The model under review builds one solid part; all positions refer to its coordinate system, in mm. Coordinates: 2 decimals unless noted, no trailing zeros. Loops run counter-clockwise (first coordinate to the right, second up) from the corner with the lowest first, then second, coordinate; pieces in that order, holes last. Notation, with made-up numbers: M 70.25,35 L 76.25,35 A19 cw 76.25,50 Z; hole C 20.25,-32 d10. An arc over 180 degrees is marked long. Write item = value, one per line. Start each with the question number.
Q1. Clearance check with flat-ended pins moving along their axes: pin 1 Ø5.5 at (x, y) = (1067.5, -9.5) entering from -Z; pin 2 Ø9 at (x, y) = (48, -6.5) entering from -Z; pin 3 Ø8 at (x, z) = (323.5, -145) entering from +Y. State where each tip first meets the part, or that it passes through.
Q2. Wall thickness on probe 1 along X at (y, z) = (-10, 0); probe 2 along Z at (x, y) = (35, -7.5); probe 3 along X at (y, z) = (-5.75, -303.5): over which ranges is each line inside the solid? List them lowest first.
Q3. Mouldability with a two-part tool opening along X and no side actions: class faces 1 (the face through (1075.143, -8.874, -470.218)), 2 (the face through (-1026.754, -8.874, -470.972)), 3 (the face through (1025.4, -8.87, -468.37)), 4 (the face through (-1074.483, -8.874, -467.698)) as released by +X, released by -X, zero draft, split by the parting line, or undercut.
Q4. We need section C-C on y = -3.25. Count the separate pieces of the cut face and the enclosed holes in it, and give its area (3 significant figures).
Q5. We need section B-B on z = -416. Give the boundary of the cut face in (x, y), and give its area (3 significant figures).
Q6. We need section A-A on x = -43. Give the boundary of the cut face in (y, z), and give its area (3 significant figures).
Q7. We need section D-D on x = 292.5. Give the boundary of the cut face in (y, z), and give its area (3 significant figures).
from build123d import *

# Parameters (mm, degrees)
F0_W     = 9
F0_H     = 432
F0_H_2   = 9
F1_DEPTH = 18


# Not quite as in the source:
# - a feature names something its author has since deleted; it is built from what else it names


with BuildPart() as f1:
    # F0 (on Front) → F1 (new body)
    with BuildSketch(Plane.XZ):
        Polygon((0, 75.8756743552), (-1100, 75.8756743552), (-1100, 66.8756743552), (-1091, 66.8756743552), (0, 66.8756743552), (1091, 66.8756743552), (1091, 75.8756743552), align=None)
        with BuildLine():
            Line((-973.3476458471, -374.1243256448), (-1054.6076226562, -374.1243256448))
            ThreePointArc((-1054.6076226562, -374.1243256448), (-1051.7483407187, -375.721921149), (-1051.265639742, -378.9614896944))
            Line((-1051.265639742, -378.9614896944), (-1098.3606008427, -558.954299013))
            ThreePointArc((-1098.3606008427, -558.954299013), (-1097.4812264988, -563.2754093644), (-1093.523436793, -565.219938755))
            Line((-1093.523436793, -565.219938755), (-1078.8076104242, -565.219938755))
            ThreePointArc((-1078.8076104242, -565.219938755), (-1076.2129629213, -564.4940239596), (-1074.371712623, -562.5270604893))
            Line((-1074.371712623, -562.5270604893), (-977.7835436484, -376.8172039105))
            ThreePointArc((-977.7835436484, -376.8172039105), (-975.94229335, -374.8502404402), (-973.3476458471, -374.1243256448))
        make_face()
        with BuildLine():
            Line((1100, 66.8756743552), (1091, 66.8756743552))
            Line((1091, 66.8756743552), (1091, -365.0378882885))
            Line((1091, -365.0378882885), (1091, -365.1243256448))
            Line((1091, -365.1243256448), (0, -365.1243256448))
            Line((0, -365.1243256448), (-1091, -365.1243256448))
            Line((-1091, -365.1243256448), (-1091, -374.1243256448))
            Line((-1091, -374.1243256448), (-1055, -374.1243256448))
            ThreePointArc((-1055, -374.1243256448), (-1054.8038113281, -374.1191399972), (-1054.6076226562, -374.1243256448))
            Line((-1054.6076226562, -374.1243256448), (-973.3476458471, -374.1243256448))
            Line((-973.3476458471, -374.1243256448), (0, -374.1243256448))
            Line((0, -374.1243256448), (973.3476458471, -374.1243256448))
            Line((973.3476458471, -374.1243256448), (1054.6076226562, -374.1243256448))
            ThreePointArc((1054.6076226562, -374.1243256448), (1054.8038113281, -374.1191399972), (1055, -374.1243256448))
            Line((1055, -374.1243256448), (1100, -374.1243256448))
            Line((1100, -374.1243256448), (1100, 66.8756743552))
        make_face()
        with Locations((-1095.5, -149.1243256448)):
            Rectangle(F0_W, F0_H)
        with Locations((-1095.5, -369.6243256448)):
            Rectangle(F0_W, F0_H_2)
        with Locations((1095.5, 71.3756743552)):
            Rectangle(F0_W, F0_H_2)
        with BuildLine():
            ThreePointArc((1051.265639742, -378.9614896944), (1051.7483407187, -375.721921149), (1054.6076226562, -374.1243256448))
            Line((1054.6076226562, -374.1243256448), (973.3476458471, -374.1243256448))
            ThreePointArc((973.3476458471, -374.1243256448), (975.94229335, -374.8502404402), (977.7835436484, -376.8172039105))
            Line((977.7835436484, -376.8172039105), (1074.371712623, -562.5270604893))
            ThreePointArc((1074.371712623, -562.5270604893), (1076.2129629213, -564.4940239596), (1078.8076104242, -565.219938755))
            Line((1078.8076104242, -565.219938755), (1093.523436793, -565.219938755))
            ThreePointArc((1093.523436793, -565.219938755), (1097.4812264988, -563.2754093644), (1098.3606008427, -558.954299013))
            Line((1098.3606008427, -558.954299013), (1051.265639742, -378.9614896944))
        make_face()
        Polygon((0, 66.8756743552), (-1091, 66.8756743552), (-1091, -365.1243256448), (0, -365.1243256448), (1091, -365.1243256448), (1091, -365.0378882885), (1091, 66.8756743552), align=None)
        with BuildLine():
            ThreePointArc((-1041, -227.1243239641), (-1037.4852813742, -218.6390425899), (-1029, -215.1243239641))
            Line((-1029, -215.1243239641), (-803, -215.1243239641))
            ThreePointArc((-803, -215.1243239641), (-794.5147186258, -218.6390425899), (-791, -227.1243239641))
            Line((-791, -227.1243239641), (-791, -303.1243256448))
            ThreePointArc((-791, -303.1243256448), (-794.5147186258, -311.609607019), (-803, -315.1243256448))
            Line((-803, -315.1243256448), (-1029, -315.1243256448))
            ThreePointArc((-1029, -315.1243256448), (-1037.4852813742, -311.609607019), (-1041, -303.1243256448))
            Line((-1041, -303.1243256448), (-1041, -227.1243239641))
        make_face(mode=Mode.SUBTRACT)
        with BuildLine():
            ThreePointArc((-118.4479668736, -227.1243239641), (-114.9332482479, -218.6390425899), (-106.4479668736, -215.1243239641))
            Line((-106.4479668736, -215.1243239641), (119.5520331264, -215.1243239641))
            ThreePointArc((119.5520331264, -215.1243239641), (128.0373145006, -218.6390425899), (131.5520331264, -227.1243239641))
            Line((131.5520331264, -227.1243239641), (131.5520331264, -303.1243256448))
            ThreePointArc((131.5520331264, -303.1243256448), (128.0373145006, -311.609607019), (119.5520331264, -315.1243256448))
            Line((119.5520331264, -315.1243256448), (-106.4479668736, -315.1243256448))
            ThreePointArc((-106.4479668736, -315.1243256448), (-114.9332482479, -311.609607019), (-118.4479668736, -303.1243256448))
            Line((-118.4479668736, -303.1243256448), (-118.4479668736, -227.1243239641))
        make_face(mode=Mode.SUBTRACT)
        with BuildLine():
            Line((791, -303.1243256448), (791, -227.1243239641))
            ThreePointArc((791, -227.1243239641), (794.5147186258, -218.6390425899), (803, -215.1243239641))
            Line((803, -215.1243239641), (1029, -215.1243239641))
            ThreePointArc((1029, -215.1243239641), (1037.4852813742, -218.6390425899), (1041, -227.1243239641))
            Line((1041, -227.1243239641), (1041, -303.1243256448))
            ThreePointArc((1041, -303.1243256448), (1037.4852813742, -311.609607019), (1029, -315.1243256448))
            Line((1029, -315.1243256448), (803, -315.1243256448))
            ThreePointArc((803, -315.1243256448), (794.5147186258, -311.609607019), (791, -303.1243256448))
        make_face(mode=Mode.SUBTRACT)
        with BuildLine():
            ThreePointArc((-1041, 4.8756749481), (-1037.4852813742, 13.3609563223), (-1029, 16.8756749481))
            Line((-1029, 16.8756749481), (-803, 16.8756749481))
            ThreePointArc((-803, 16.8756749481), (-794.5147186258, 13.3609563223), (-791, 4.8756749481))
            Line((-791, 4.8756749481), (-791, -21.1243239343))
            ThreePointArc((-791, -21.1243239343), (-794.5147186258, -29.6096053086), (-803, -33.1243239343))
            Line((-803, -33.1243239343), (-1029, -33.1243239343))
            ThreePointArc((-1029, -33.1243239343), (-1037.4852813742, -29.6096053086), (-1041, -21.1243239343))
            Line((-1041, -21.1243239343), (-1041, 4.8756749481))
        make_face(mode=Mode.SUBTRACT)
        with BuildLine():
            ThreePointArc((-118.4479668736, 4.8756749481), (-114.9332482479, 13.3609563223), (-106.4479668736, 16.8756749481))
            Line((-106.4479668736, 16.8756749481), (119.5520331264, 16.8756749481))
            ThreePointArc((119.5520331264, 16.8756749481), (128.0373145006, 13.3609563223), (131.5520331264, 4.8756749481))
            Line((131.5520331264, 4.8756749481), (131.5520331264, -21.1243239343))
            ThreePointArc((131.5520331264, -21.1243239343), (128.0373145006, -29.6096053086), (119.5520331264, -33.1243239343))
            Line((119.5520331264, -33.1243239343), (-106.4479668736, -33.1243239343))
            ThreePointArc((-106.4479668736, -33.1243239343), (-114.9332482479, -29.6096053086), (-118.4479668736, -21.1243239343))
            Line((-118.4479668736, -21.1243239343), (-118.4479668736, 4.8756749481))
        make_face(mode=Mode.SUBTRACT)
        with BuildLine():
            Line((803, 16.8756749481), (1029, 16.8756749481))
            ThreePointArc((1029, 16.8756749481), (1037.4852813742, 13.3609563223), (1041, 4.8756749481))
            Line((1041, 4.8756749481), (1041, -21.1243239343))
            ThreePointArc((1041, -21.1243239343), (1037.4852813742, -29.6096053086), (1029, -33.1243239343))
            Line((1029, -33.1243239343), (803, -33.1243239343))
            ThreePointArc((803, -33.1243239343), (794.5147186258, -29.6096053086), (791, -21.1243239343))
            Line((791, -21.1243239343), (791, 4.8756749481))
            ThreePointArc((791, 4.8756749481), (794.5147186258, 13.3609563223), (803, 16.8756749481))
        make_face(mode=Mode.SUBTRACT)
    extrude(amount=F1_DEPTH)


solid = f1.part
Returned:
q1.pin_1 = -554.6
q1.pin_2 = -374.12
q1.pin_3 = 0
q2.probe_1 = -1100 to -1041, -791 to -118.45, 131.55 to 791, 1041 to 1100
q2.probe_2 = -374.12 to -315.12, -215.12 to -33.12, 16.88 to 75.88
q2.probe_3 = -1100 to -1040.99, -791.01 to -118.44, 131.55 to 791.01, 1040.99 to 1100
q3.face_1 = released by +X
q3.face_2 = undercut
q3.face_3 = undercut
q3.face_4 = released by -X
q4.separate_pieces = 1
q4.enclosed_holes = 6
q4.area = 897,000 mm^2
q5.outline = M -1060.96,-18 L -998.16,-18 L -998.16,0 L -1060.96,0 Z; M 998.16,-18 L 1060.96,-18 L 1060.96,0 L 998.16,0 Z
q5.area = 2,260 mm^2
q6.outline = M -18,-374.12 L 0,-374.12 L 0,-315.12 L -18,-315.12 Z; M -18,-215.12 L 0,-215.12 L 0,-33.12 L -18,-33.12 Z; M -18,16.88 L 0,16.88 L 0,75.88 L -18,75.88 Z
q6.area = 5,400 mm^2
q7.outline = M -18,-374.12 L 0,-374.12 L 0,75.88 L -18,75.88 Z
q7.area = 8,100 mm^2
